Could you check a few things on this model? Use its own coordinates, in mm. Face numbers are marked on the shaded views. A direction names the side the tool comes from. Round coordinates to 2 decimals unless told otherwise and drop trailing zeros. Write each loop counter-clockwise with the first axis right and the second up, starting at its lowest first coordinate (ties: lowest second). Pieces come first, ordered by that corner, then holes. Notation, with made-up numbers: M 43,25 L 81,25 A30 ccw 81,55 Z; hole C 37,56 d10. An arc over 180 degrees is marked long. One line per item, written item: value. Start each with the question number.
(1) I want a section at A-A on x = 5. Please give me the cut outline in (y, z), and give its area (3 significant figures).
(2) I want a section at B-B on y = 40. Please give me the cut outline in (x, z).
(3) I want a section at D-D on z = 22. Please give me the cut outline in (x, y).
(4) Which directions (+Z, -Z, +X, -X, +Y, -Y) give clear straight access to the entire face, cutting with the end or side of a thin tool? Please do the marked faces 1, 2 and 3.
(5) I'm going to push flat-ended pins straight in: pin 1 Ø1 at (x, z) = (8, 8) entering from -Y; pin 2 Ø3.5 at (x, y) = (5, 40) entering from -Z; pin 3 Ø2.5 at (x, y) = (5, -40) entering from +Z; pin 4 Ø5 at (x, y) = (3, 31.5) entering from +Z. Where does each tip first touch, or does it pass through?
(6) If I drill on L1, parallel to Y at x = 5, z = 1.4; L2, parallel to Y at x = 5, z = 2.3; L3, parallel to Z at x = 4.5, y = 45.5, over which ranges is the centre line in solid material (lowest first)?
(7) I want a section at C-C on z = 7.75. Please give me the cut outline in (x, y), and give its area (3 significant figures).
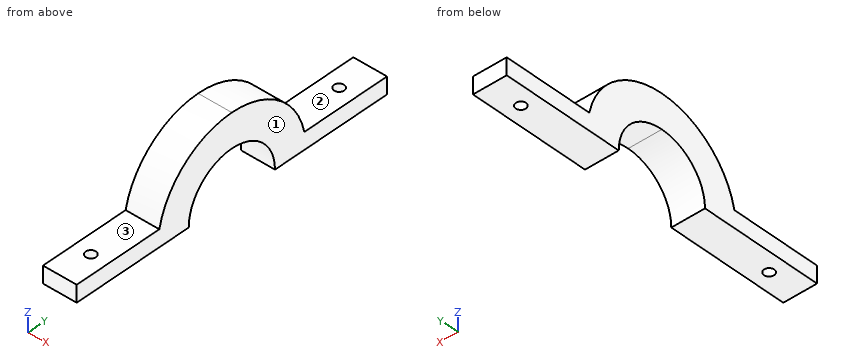
```python
from build123d import *

# Parameters (mm, degrees)
F1_DEPTH = 10
F2_R     = 1.5
F3_DEPTH = 25


with BuildPart() as f1:
    # F0 (on Right) → F1 (new body)
    with BuildSketch(Plane.YZ):
        with BuildLine():
            ThreePointArc((-13.9, 0), (-9.828784, 9.828784), (0, 13.9))
            ThreePointArc((0, 13.9), (9.828784, 9.828784), (13.9, 0))
            Line((13.9, 0), (50, 0))
            Line((50, 0), (50, 5))
            Line((50, 5), (23.371136, 5))
            ThreePointArc((23.371136, 5), (15.028473, 18.583729), (0, 23.9))
            ThreePointArc((0, 23.9), (-15.028473, 18.583729), (-23.371136, 5))
            Line((-23.371136, 5), (-50, 5))
            Line((-50, 5), (-50, 0))
            Line((-50, 0), (-13.9, 0))
        make_face()
    extrude(amount=F1_DEPTH)

    # F2 (on face) → F3 (cut)
    with BuildSketch(Plane.XY.offset(5)):
        with Locations((5, 40)):
            Circle(F2_R)
        with Locations((5, -40)):
            Circle(F2_R)
    extrude(amount=-F3_DEPTH, mode=Mode.SUBTRACT)


solid = f1.part
```
Found:
1. outline: M -50,0 L -41.5,0 L -41.5,5 L -50,5 Z; M -38.5,0 L -13.9,0 A13.9 cw 0,13.9 A13.9 cw 13.9,0 L 38.5,0 L 38.5,5 L 23.37,5 A23.9 ccw 0,23.9 A23.9 ccw -23.37,5 L -38.5,5 Z; M 41.5,0 L 50,0 L 50,5 L 41.5,5 Z
1. area: 827 mm²
2. outline: M 0,0 L 3.5,0 L 3.5,5 L 0,5 Z; M 6.5,0 L 10,0 L 10,5 L 6.5,5 Z
3. outline: M 0,-9.34 L 10,-9.34 L 10,9.34 L 0,9.34 Z
4. face 1: +Z, -Z, +X, +Y, -Y
4. face 2: +Z, +X, -X, +Y
4. face 3: +Z, +X, -X, -Y
5. pin 1: stops at y = -22.69
5. pin 2: stops at z = 0
5. pin 3: passes through
5. pin 4: stops at z = 5
6. L1: y = -50 to -41.5, -38.5 to -13.83, 13.83 to 38.5, 41.5 to 50
6. L2: y = -50 to -41.5, -38.5 to -13.71, 13.71 to 38.5, 41.5 to 50
6. L3: z = 0 to 5
7. outline: M 0,-22.61 L 10,-22.61 L 10,-11.54 L 0,-11.54 Z; M 0,11.54 L 10,11.54 L 10,22.61 L 0,22.61 Z
7. area: 221 mm²
